```python
from build123d import *

# Parameters (mm, degrees)
SKETCH1_R           = 2.125
BOSS_EXTRUDE1_DEPTH = 2.5
SKETCH2_W           = 15
SKETCH2_H           = 8
BOSS_EXTRUDE2_DEPTH = 8
CUT_EXTRUDE1_REACH  = 29.5
SKETCH4_R           = 2
SKETCH6_W           = 7.25
SKETCH6_H           = 3.25
CUT_EXTRUDE2_DEPTH  = 11.5


with BuildPart() as part:
    # Sketch1 → Boss-Extrude1 (new body)
    with BuildSketch(Plane.XY):
        with BuildLine():
            Line((2.5, 10), (2.5, 30))
            Line((2.5, 30), (17.5, 30))
            Line((17.5, 30), (17.5, 10))
            ThreePointArc((17.5, 10), (10, 2.5), (2.5, 10))
        make_face()
        with Locations((10, 10)):
            Circle(SKETCH1_R, mode=Mode.SUBTRACT)
    boss_extrude1 = extrude(amount=BOSS_EXTRUDE1_DEPTH)

    # Sketch2 → Boss-Extrude2 (add)
    with BuildSketch(Plane(origin=(0, 0, 0), x_dir=(-1, 0, 0), z_dir=(0, 0, -1))):
        with Locations((-10, 26)):
            Rectangle(SKETCH2_W, SKETCH2_H)
    extrude(amount=BOSS_EXTRUDE2_DEPTH)

    # Mirror1: Boss-Extrude1 across plane
    add(boss_extrude1.mirror(Plane.XY.offset(-4)))

    # Sketch4 → Cut-Extrude1 (cut, up to next)
    with BuildSketch(Plane(origin=(0, 30, 0), x_dir=(1, 0, 0), z_dir=(0, 1, 0)), mode=Mode.PRIVATE) as cut_extrude1_sk1:
        with Locations((10, 4)):
            Circle(SKETCH4_R)
    cut_extrude1_tool1 = extrude(cut_extrude1_sk1.sketch, amount=-CUT_EXTRUDE1_REACH, mode=Mode.PRIVATE) & part.part
    add(cut_extrude1_tool1.solids().sort_by_distance((10, 30, -4))[0], mode=Mode.SUBTRACT)

    # Sketch6 → Cut-Extrude2 (cut)
    with BuildSketch(Plane.ZY.offset(-2.5)):
        with Locations((-4, 25.975)):
            Rectangle(SKETCH6_W, SKETCH6_H)
    extrude(amount=-CUT_EXTRUDE2_DEPTH, mode=Mode.SUBTRACT)


solid = part.part
```
Check sheet for the modelled part. Datum: model origin and axes. Units: mm. A direction names the side the tool comes from. Round coordinates to 2 decimals unless told otherwise and drop trailing zeros. Order: outer loops, then holes, each group sorted by start corner. A loop starts at its lowest first (then second) coordinate and runs counter-clockwise, first axis right, second up. Notation, with made-up numbers: (46.25, 0) - (72.25, 0) arc R16 ccw to (72.25, 5) - close; hole circle Ø3 at (82, -32.5). An arc over 180 degrees is marked (long way). Write item = value, one per line.
Q1. Go/stop test with a flat-tipped pin: pin 1 (5 mm diameter, centred on x = 16, z = -5, fed in from -Y). Record where the tip stops, or that it passes through.
Computed:
pin_1 = 22
Q2. Section check D-D (z = -1.5). Record the boundary of the cut face in (x, y), and give its area (3 significant figures).
Computed:
outline = (2.5, 22) - (17.5, 22) - (17.5, 30) - (2.5, 30) - (2.5, 27.6) - (14, 27.6) - (14, 24.35) - (2.5, 24.35) - close
area = 82.6 mm^2
Q3. Section check B-B (y = 26). Record the boundary of the cut face in (x, z) (3 decimals).
Computed:
outline = (2.5, -10.5) - (17.5, -10.5) - (17.5, 2.5) - (2.5, 2.5) - (2.5, -0.375) - (14, -0.375) - (14, -7.625) - (2.5, -7.625) - close
Q4. Draft check along Z on faces 4 (the face through (8.31, 8.71, 1.23)), 5 (the face through (8, 27.6, -5)), 6 (the face through (8, 26, -7.625)), 7 (the face through (10, 16, -10.5)). Enter one of: pulls with the +Z half, pulls with the -Z half, needs draft (parallel to the pull), parting line crosses it, or undercut.
Computed:
face_4 = needs draft
face_5 = undercut
face_6 = undercut
face_7 = pulls with the -Z half
Q5. Thickness scan on line 1 along Y through (x, z) = (11.25, -2.25); line 2 along Y through (x, z) = (10, -8.65) (3 decimals); line 3 along Z through (x, y) = (14.25, 15.25). Record the ranges inside material, lowest first.
Computed:
line_1 = 22 to 24.35, 27.6 to 30
line_2 = 2.5 to 7.875, 12.125 to 30
line_3 = -10.5 to -8, 0 to 2.5
Q6. Section check C-C (z = -4). Record the boundary of the cut face in (x, y), and give its area (3 significant figures).
Computed:
outline = (2.5, 22) - (8, 22) - (8, 24.35) - (2.5, 24.35) - close; (2.5, 27.6) - (8, 27.6) - (8, 30) - (2.5, 30) - close; (12, 22) - (17.5, 22) - (17.5, 30) - (12, 30) - (12, 27.6) - (14, 27.6) - (14, 24.35) - (12, 24.35) - close
area = 63.6 mm^2
Q7. Section check A-A (x = 10). Record the boundary of the cut face in (y, z) (3 decimals).
Computed:
outline = (2.5, -10.5) - (7.875, -10.5) - (7.875, -8) - (2.5, -8) - close; (2.5, 0) - (7.875, 0) - (7.875, 2.5) - (2.5, 2.5) - close; (12.125, -10.5) - (30, -10.5) - (30, -6) - (27.6, -6) - (27.6, -7.625) - (24.35, -7.625) - (24.35, -6) - (22, -6) - (22, -8) - (12.125, -8) - close; (12.125, 0) - (22, 0) - (22, -2) - (24.35, -2) - (24.35, -0.375) - (27.6, -0.375) - (27.6, -2) - (30, -2) - (30, 2.5) - (12.125, 2.5) - close
Q8. Tool access check on faces 1 (the face through (10, 23, -2)), 2 (the face through (8, 26, -0.375)), 3 (the face through (10.1, 12.4, 0)). Record the directions out of +Z, -Z, +X, -X, +Y, -Y that give a thin tool (end or side, any length) a straight path to the whole face; none if there is none.
Computed:
face_1 = +Y, -Y
face_2 = -X
face_3 = +X, -X, -Y
